The model under review builds one solid part; all positions refer to its coordinate system, in mm. Face numbers are marked on the shaded views. A direction names the side the tool comes from. Give positions to 0.01 mm unless a question says otherwise; leave off trailing zeros. Write each loop counter-clockwise with the first axis right and the second up, starting at its lowest first coordinate (ties: lowest second). Pieces come first, ordered by that corner, then holes. Notation, with made-up numbers: (0, -40) - (11, -40) arc R29 ccw to (11, -2) - close; hole circle Ø3 at (-34, 73.5). An arc over 180 degrees is marked (long way). Write item = value, one per line.
```python
from build123d import *

# Parameters (mm, degrees)
SKIZZE1_R                       = 20
AUFSATZ_LINEAR_AUSTRAGEN1_DEPTH = 7
SKIZZE3_R                       = 12.875
AUFSATZ_LINEAR_AUSTRAGEN2_DEPTH = 7
SKIZZE7_W                       = 15
SKIZZE7_H                       = 20
AUFSATZ_LINEAR_AUSTRAGEN3_DEPTH = 10
SKIZZE8_R                       = 5
SCHNITT_LINEAR_AUSTRAGEN2_DEPTH = 7
VERRUNDUNG2_R                   = 1
SCHNITT_LINEAR_START            = -3
SKIZZE9_R                       = 5
SCHNITT_LINEAR_AUSTRAGEN3_DEPTH = 3
SKIZZE5_R                       = 3.5
SCHNITT_LINEAR_AUSTRAGEN4_DEPTH = 5


with BuildPart() as part:
    # Skizze1 → Aufsatz-Linear austragen1 (new body)
    with BuildSketch(Plane(origin=(0, 0, 0), x_dir=(1, 0, 0), z_dir=(0, 1, 0))):
        with Locations(Location((0, 0, 0), (0, 0, 270))):
            Circle(SKIZZE1_R)
    extrude(amount=AUFSATZ_LINEAR_AUSTRAGEN1_DEPTH)

    # Skizze3 → Aufsatz-Linear austragen2 (add)
    with BuildSketch(Plane(origin=(0, 7, 0), x_dir=(1, 0, 0), z_dir=(0, 1, 0))):
        with Locations(Location((0, 0, 0), (0, 0, 270))):
            Circle(SKIZZE3_R)
    extrude(amount=AUFSATZ_LINEAR_AUSTRAGEN2_DEPTH)

    # Skizze7 → Aufsatz-Linear austragen3 (add)
    with BuildSketch(Plane(origin=(0, 14, 0), x_dir=(1, 0, 0), z_dir=(0, 1, 0))):
        Rectangle(SKIZZE7_W, SKIZZE7_H)
    extrude(amount=AUFSATZ_LINEAR_AUSTRAGEN3_DEPTH)

    # Skizze8 → Schnitt-Linear austragen2 (cut)
    with BuildSketch(Plane(origin=(0, 24, 0), x_dir=(1, 0, 0), z_dir=(0, 1, 0))):
        with Locations(Location((0, 0, 0), (0, 0, 270))):
            Circle(SKIZZE8_R)
    extrude(amount=-SCHNITT_LINEAR_AUSTRAGEN2_DEPTH, mode=Mode.SUBTRACT)

    # Verrundung2
    verrundung2_edges = [part.edges().sort_by_distance(p)[0] for p in [
        (0, 24, -5),
    ]]
    fillet(verrundung2_edges, radius=VERRUNDUNG2_R)

    # Skizze9 → Schnitt-Linear austragen3 (cut)
    with BuildSketch(Plane.XZ.offset(SCHNITT_LINEAR_START)):
        with Locations(Location((0, 0, 0), (0, 0, 90))):
            Circle(SKIZZE9_R)
    extrude(amount=SCHNITT_LINEAR_AUSTRAGEN3_DEPTH, mode=Mode.SUBTRACT)

    # Skizze5 → Schnitt-Linear austragen4 (cut)
    with BuildSketch(Plane(origin=(0, 0, 0), x_dir=(-1, 0, 0), z_dir=(0, -1, 0))):
        with Locations(Location((0, -15, 0), (0, 0, 90))):
            Circle(SKIZZE5_R)
        with Locations(Location((-12.990381057, 7.5, 0), (0, 0, 90))):
            Circle(SKIZZE5_R)
        with Locations(Location((12.990381057, 7.5, 0), (0, 0, 90))):
            Circle(SKIZZE5_R)
    extrude(amount=-SCHNITT_LINEAR_AUSTRAGEN4_DEPTH, mode=Mode.SUBTRACT)


solid = part.part
```
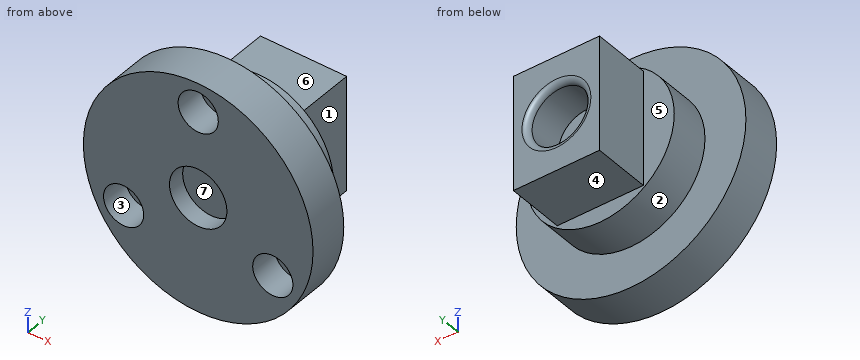
1. Take a section at B-B on z = -9. Give the boundary of the cut face in (x, y).
Findings below:
outline = (-17.86, 0) - (-16.15, 0) - (-16.15, 5) - (-9.83, 5) - (-9.83, 0) - (9.83, 0) - (9.83, 5) - (16.15, 5) - (16.15, 0) - (17.86, 0) - (17.86, 7) - (9.21, 7) - (9.21, 14) - (7.5, 14) - (7.5, 24) - (-7.5, 24) - (-7.5, 14) - (-9.21, 14) - (-9.21, 7) - (-17.86, 7) - close
2. For line 1 (X direction, y = 2.25, z = 0); line 2 (X direction, y = 3.1, z = -7.5); line 3 (X direction, y = 18.5, z = -7.5), list the stretches that pass through material, from the lowest coordinate up. Write a range as from..to.
Findings below:
line_1 = -20..-5, 5..20
line_2 = -18.54..-16.49, -9.49..9.49, 16.49..18.54
line_3 = -7.5..7.5
3. Draft analysis for pull direction Z (two halves, no side actions). For the marked faces 5, 6 and 7, state which applies: +Z half, -Z half, draft (parallel to the pull), parting line (faces both ways), or undercut.
Findings below:
face_5 = draft
face_6 = +Z half
face_7 = undercut
4. Insertion check: P1, Ø3, axis at y = 3.5, z = -7, coming from the +X side; P2, Ø4, axis at x = -12.99, z = -7.5, coming from the +Y side; P3, Ø5, axis at x = 2, z = 1, coming from the +Y side; P4, Ø1, axis at y = 19.5, z = -12, coming from the +X side. Each pin has a flat end and moves straight along its axis. Give the tip position at first contact, or say it passes through.
Findings below:
P1 = 19.23
P2 = 7
P3 = 17
P4 = through
5. Take a section at A-A on x = 0. Give the boundary of the cut face in (y, z) (3 decimals).
Findings below:
outline = (0, -20) - (7, -20) - (7, -12.875) - (14, -12.875) - (14, -10) - (24, -10) - (24, -6) arc R1 ccw to (23, -5) - (17, -5) - (17, 5) - (23, 5) arc R1 ccw to (24, 6) - (24, 10) - (14, 10) - (14, 12.875) - (7, 12.875) - (7, 20) - (0, 20) - (0, 18.5) - (5, 18.5) - (5, 11.5) - (0, 11.5) - (0, 5) - (3, 5) - (3, -5) - (0, -5) - close
6. Take a section at D-D on z = 0. Give the boundary of the cut face in (x, y) (3 decimals).
Findings below:
outline = (-20, 0) - (-5, 0) - (-5, 3) - (5, 3) - (5, 0) - (20, 0) - (20, 7) - (12.875, 7) - (12.875, 14) - (7.5, 14) - (7.5, 24) - (6, 24) arc R1 ccw to (5, 23) - (5, 17) - (-5, 17) - (-5, 23) arc R1 ccw to (-6, 24) - (-7.5, 24) - (-7.5, 14) - (-12.875, 14) - (-12.875, 7) - (-20, 7) - close
7. Machinability: for the marked faces 1, 2, 3 and 4, which of the approach directions +Z, -Z, +X, -X, +Y, -Y give a long, thin tool a straight path to every point of the face, cutting with its end or side? Answer none if there is none.
Findings below:
face_1 = +Z, -Z, +X, +Y
face_2 = +Y
face_3 = -Y
face_4 = -Z, +X, -X, +Y
8. Take a section at C-C on y = 15.5. Give the boundary of the cut face in (x, z), and give its area (3 significant figures).
Findings below:
outline = (-7.5, -10) - (7.5, -10) - (7.5, 10) - (-7.5, 10) - close
area = 300 mm²
